Autodesk Fusion 360 part; units mm, degrees
sketch "Roller_Insert" plane through (0, 0, 0) normal (0, 0, 1) x (1, 0, 0)
  circle A0 centre (0, 0) radius 34.925
  dimension "d1" = 69.85
extrude "Extrude2" add sketch "Roller_Insert" along normal blind 12.7
sketch "Pipe Cutout" plane through (0, 0, 12.7) normal (0, 0, 1) x (-1, 0, 0)
  circle A0 centre (0, 0) radius 34.925
  circle A1 centre (0, 0) radius 6.45
  dimension "d9" = 12.9
extrude "Extrude3" cut sketch "Pipe Cutout" against normal through all contours A1
chamfer "Chamfer1" distance 2 angle 45 4 edges at (6.0135, -2.3324, 12.7) (-32.5615, -12.6294, 12.7) (-32.5615, -12.6294, 0) (6.0135, 2.3324, 0)
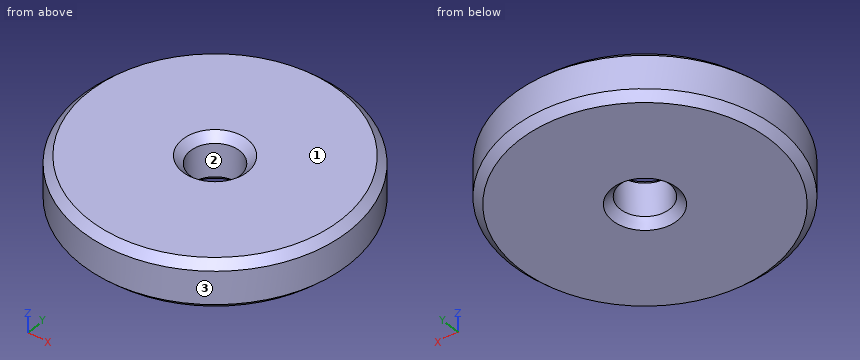
Here's how the part is built. I have some questions about the finished solid (model axes, mm). Face numbers are marked on the shaded views. Round coordinates to 2 decimals unless told otherwise and drop trailing zeros. Loops run counter-clockwise (first coordinate to the right, second up) from the corner with the lowest first, then second, coordinate; pieces in that order, holes last. Notation, with made-up numbers: (2, 24) - (12, 24) arc R35 cw to (12, 62) - close; hole circle Ø3 at (51.25, 83.25). An arc over 180 degrees is marked (long way). One line per question, with ' | ' between items. Start each with the question number.
Q1. Will these pins go through, and if not, where does the flat tip stop? pin 1 (1 mm diameter, centred on x = -21, z = 5, fed in from -Y); pin 2 (10.5 mm diameter, centred on x = 0, y = 0, fed in from +Z); pin 3 (2 mm diameter, centred on x = -18.5, y = -21, fed in from -Z); pin 4 (6 mm diameter, centred on y = 19, z = 1.5, fed in from -X).
Q2. Please list where these lines run through material, in increasing order: line 1 (Y direction, x = 0, z = 4) (3 decimals); line 2 (X direction, y = -6, z = 1); line 3 (Y direction, x = -21, z = 7). Write a range as [from, to].
Q3. I want a section at C-C (z = 5.5). Write out the boundary of the cut face in (x, y) (3 decimals), then the cut area to 3 significant figures.
Q4. I want a section at A-A (x = 0). Write out the boundary of the cut face in (y, z) (3 decimals).
Q5. We'd pull the mould along X, two halves only. Please class the marked faces 1, 2 and 3: +X half, -X half, draft (parallel to the pull), parting line (faces both ways), or undercut.
Response values:
1) pin 1: stops at y = -28.28 | pin 2: passes through | pin 3: stops at z = 0 | pin 4: stops at x = -31.02
2) line 1: y = [-34.925, -6.45], [6.45, 34.925] | line 2: x = [-33.39, -4.42], [4.42, 33.39] | line 3: y = [-27.91, 27.91]
3) outline: circle Ø69.85 at (0, 0); hole circle Ø12.9 at (0, 0) | area: 3,700 mm²
4) outline: (-34.925, 2) - (-32.925, 0) - (-8.45, 0) - (-6.45, 2) - (-6.45, 10.7) - (-8.45, 12.7) - (-32.925, 12.7) - (-34.925, 10.7) - close; (6.45, 2) - (8.45, 0) - (32.925, 0) - (34.925, 2) - (34.925, 10.7) - (32.925, 12.7) - (8.45, 12.7) - (6.45, 10.7) - close
5) face 1: draft | face 2: undercut | face 3: parting line
